Source: three-view drawing plus pictorial views. Frame: mm from the lowest corner of the part. A direction names the side the tool comes from. Round coordinates to 2 decimals unless told otherwise and drop trailing zeros. Write each loop counter-clockwise with the first axis right and the second up, starting at its lowest first coordinate (ties: lowest second). Pieces come first, ordered by that corner, then holes. Notation, with made-up numbers: (-8, 52.5) -> (45, 52.5) arc R20 cw to (45, 82.5) -> close; hole circle Ø8 at (66, -21). An arc over 180 degrees is marked (long way). Put each result on its own line as item: value.
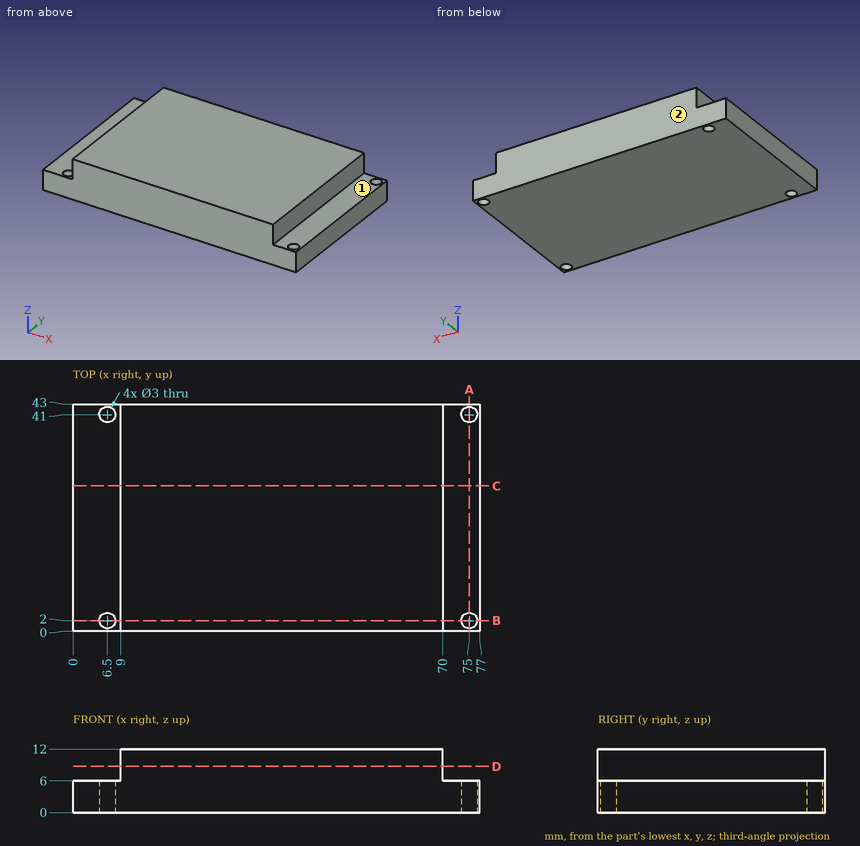
Q1. Cut plane B-B on y = 2. Output: boundary loops of the cut face in (x, z), and give its area (3 significant figures).
Ans:
outline: (0, 0) -> (5, 0) -> (5, 6) -> (0, 6) -> close; (8, 0) -> (73.5, 0) -> (73.5, 6) -> (70, 6) -> (70, 12) -> (9, 12) -> (9, 6) -> (8, 6) -> close; (76.5, 0) -> (77, 0) -> (77, 6) -> (76.5, 6) -> close
area: 792 mm^2
Q2. Cut plane D-D on z = 8.75. Output: boundary loops of the cut face in (x, y), and give its area (3 significant figures).
Ans:
outline: (9, 0) -> (70, 0) -> (70, 43) -> (9, 43) -> close
area: 2,620 mm^2
Q3. Material intervals for line 1 (X direction, y = 2, z = 2.65); line 2 (Y direction, x = 75, z = 3.3); line 3 (X direction, y = 10, z = 9.5), sorted ascending. Write a range as [from, to].
Ans:
line 1: x = [0, 5], [8, 73.5], [76.5, 77]
line 2: y = [0, 0.5], [3.5, 39.5], [42.5, 43]
line 3: x = [9, 70]
Q4. Pin query (flat end, axial travel): pin 1 (4.5 mm diameter, centred on x = 5.5, y = 13.5, fed in from +Z); pin 2 (2 mm diameter, centred on y = 29.5, z = 10, fed in from -X); pin 3 (5 mm diameter, centred on y = 31, z = 10.5, fed in from +X). Return the tip coordinate at first contact, or that it passes through.
Ans:
pin 1: stops at z = 6
pin 2: stops at x = 9
pin 3: stops at x = 70
Q5. Cut plane C-C on y = 27.5. Output: boundary loops of the cut face in (x, z), and give its area (3 significant figures).
Ans:
outline: (0, 0) -> (77, 0) -> (77, 6) -> (70, 6) -> (70, 12) -> (9, 12) -> (9, 6) -> (0, 6) -> close
area: 828 mm^2
Q6. Reachability of the marked faces 1 and 2 from +Z, -Z, +X, -X, +Y, -Y: full face, straight path, thin tool, end or side. Return the list, or none.
Ans:
face 1: +Z, +X, +Y, -Y
face 2: +Z, -Z, +X, -X, +Y
Q7. Cut plane A-A on x = 75. Output: boundary loops of the cut face in (y, z).
Ans:
outline: (0, 0) -> (0.5, 0) -> (0.5, 6) -> (0, 6) -> close; (3.5, 0) -> (39.5, 0) -> (39.5, 6) -> (3.5, 6) -> close; (42.5, 0) -> (43, 0) -> (43, 6) -> (42.5, 6) -> close
